Input: dimensioned drawing with shaded views. Units: mm. Origin: part minimum x, y, z. Coordinates: 2 decimals unless noted, no trailing zeros. Loops run counter-clockwise (first coordinate to the right, second up) from the corner with the lowest first, then second, coordinate; pieces in that order, holes last. Notation, with made-up numbers: M -6,78.25 L 31,78.25 A33 ccw 31,116.25 Z; hole C -26.75,62 d8. An arc over 180 degrees is marked long. Write item = value, one per line. Start each with the question number.
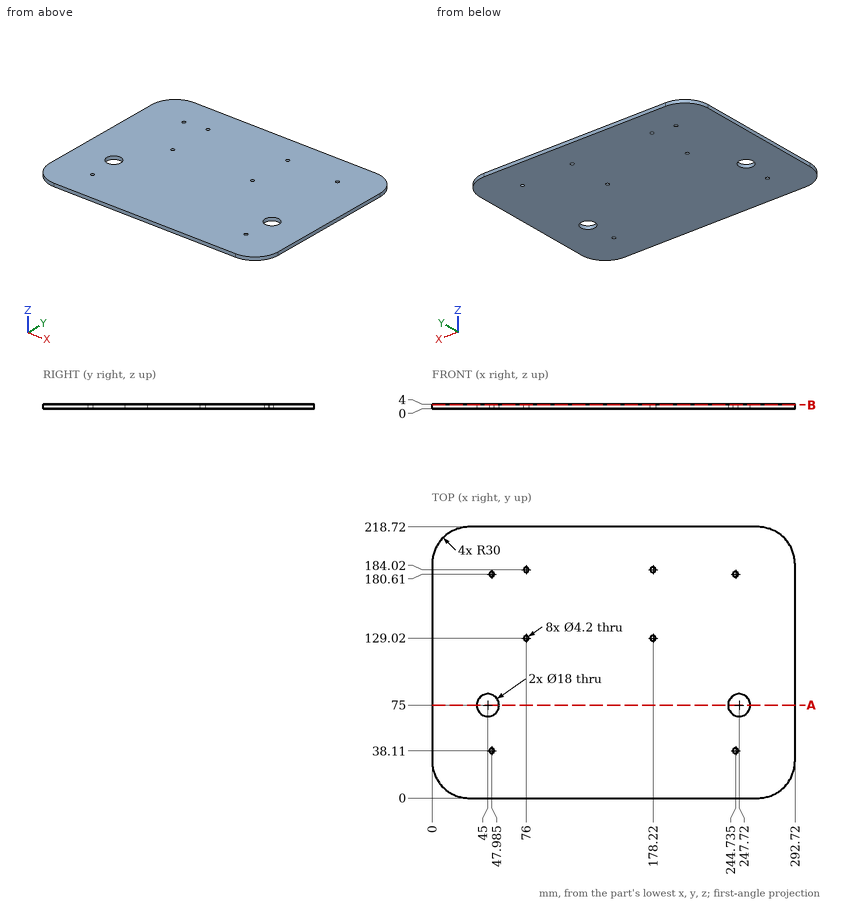
Item 1: Line query: line 1 (Y direction, x = 76, z = 1.2); line 2 (X direction, y = 75.5, z = 1.05); line 3 (Y direction, x = 76.5, z = 1.35). Output: solid intervals per line, ascending. Write a range as from..to.
Item 2: Section query A-A (y = 75). Return the cut outline in (x, z), plus the area to 3 significant figures.
Item 3: Section query B-B (z = 3.35). Count the separate pieces of the cut face and the enclosed holes in it, plus the area to 3 significant figures.
Verdict:
q1.line_1 = 0..126.92, 131.12..181.92, 186.12..218.72
q1.line_2 = 0..36.01, 53.99..238.73, 256.71..292.72
q1.line_3 = 0..126.98, 131.06..181.98, 186.06..218.72
q2.outline = M 0,0 L 36,0 L 36,4 L 0,4 Z; M 54,0 L 238.72,0 L 238.72,4 L 54,4 Z; M 256.72,0 L 292.72,0 L 292.72,4 L 256.72,4 Z
q2.area = 1,030 mm2
q3.separate_pieces = 1
q3.enclosed_holes = 10
q3.area = 62,600 mm2
